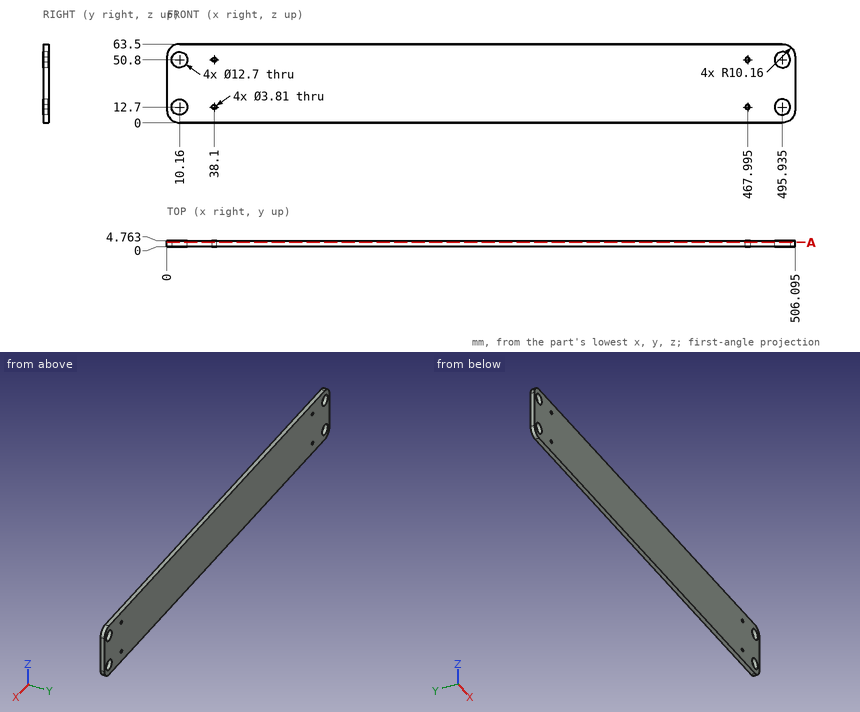
Can you work these out from the drawing? Everything is in mm from the part's minimum corner. Give positions to 0.01 mm unless a question says otherwise; leave off trailing zeros. Use a Markdown table: item, result. Add a question column.
1. I need wall thicknesses on probe 1 along X at (y, z) = (2.6, 12.7) (1 decimal); probe 2 along Z at (x, y) = (10.16, 3.3); probe 3 along X at (y, z) = (4.55, 16) (1 decimal). Which ranges of each line are inside material? Lowest first, please. Write a range as from..to.
2. Suppose I cut it at A-A (y = 3.5). Give the number of separate pieces and of enclosed holes in the cut face, and give its area (3 significant figures).
3. For pin 1 Ø11.5 at (x, z) = (495.935, 12.7) entering from +Y, with a flat end and sliding along its axis, tell me the tip position at first contact or that it passes through.
Results list:
| question | item | result |
|---|---|---|
| 1 | probe 1 | x = 0..3.8, 16.5..36.2, 40..466.1, 469.9..489.6, 502.3..506.1 |
| 1 | probe 2 | z = 0..6.35, 19.05..44.45, 57.15..63.5 |
| 1 | probe 3 | x = 0..4.7, 15.6..490.5, 501.4..506.1 |
| 2 | separate pieces | 1 |
| 2 | enclosed holes | 8 |
| 2 | area | 31,500 mm² |
| 3 | pin 1 | passes through |
